```python
from build123d import *

# Parameters (mm, degrees)
SKETCH1_W             = 168
SKETCH1_H             = 89
BOSS_EXTRUDE1_DEPTH   = 70
SHELL1_T              = -0.8
F_8_0MM_DOWEL_HOLE1_D = 8


with BuildPart() as part:
    # Sketch1 → Boss-Extrude1 (new body)
    with BuildSketch(Plane(origin=(0, 0, 0), x_dir=(1, 0, 0), z_dir=(0, 1, 0))):
        Rectangle(SKETCH1_W, SKETCH1_H)
    extrude(amount=BOSS_EXTRUDE1_DEPTH)

    # Shell1
    shell1_openings = [part.faces().sort_by_distance(p)[0] for p in [
        (84, 35, 0),
    ]]
    offset(amount=SHELL1_T, openings=shell1_openings, kind=Kind.INTERSECTION)

    # Ø8.0mm Dowel Hole1 (through all)
    with Locations(Plane.XY.offset(44.5)):
        with Locations((64, 10), (-74, 60), (-64, 47.5), (-74, 35), (-64, 22.5), (-74, 10), (-54.285714286, 60), (-44.285714286, 47.5), (-54.285714286, 35), (-44.285714286, 22.5), (-54.285714286, 10), (-34.571428571, 60), (-24.571428571, 47.5), (-34.571428571, 35), (-24.571428571, 22.5), (-34.571428571, 10), (-14.857142857, 60), (-4.857142857, 47.5), (-14.857142857, 35), (-4.857142857, 22.5), (-14.857142857, 10), (4.857142857, 60), (14.857142857, 47.5), (4.857142857, 35), (14.857142857, 22.5), (4.857142857, 10), (24.571428571, 60), (34.571428571, 47.5), (24.571428571, 35), (34.571428571, 22.5), (24.571428571, 10), (44.285714286, 60), (54.285714286, 47.5), (44.285714286, 35), (54.285714286, 22.5), (44.285714286, 10), (64, 60), (74, 47.5), (64, 35), (74, 22.5)):
            Hole(F_8_0MM_DOWEL_HOLE1_D / 2)


solid = part.part
```
Can you work these out from the model? Positions are in its coordinate system, mm. A direction names the side the tool comes from. Coordinates: 2 decimals unless noted, no trailing zeros. Order: outer loops, then holes, each group sorted by start corner. A loop starts at its lowest first (then second) coordinate and runs counter-clockwise, first axis right, second up.
1. If we section it at B-B (x = 64): Give the number of separate pieces and of enclosed holes in the cut face, then the cut area to 3 significant figures.
2. For faces 1 (the face through (-73.479, 38.966, -44.106)), 2 (the face through (-83.2, 35, 1)), which set-ups out of +Z, -Z, +X, -X, +Y, -Y let a thin tool reach every point of the face, with its end or its side?
3. Thinking about a two-plate mould opening in Y: for faces 3 (the face through (-1, 70, -1)), 4 (the face through (-33.704, 56.095, 44.094)), which applies, +Y half, -Y half, draft (parallel to the pull), parting line (faces both ways), or undercut?
4. I'm going to push flat-ended pins straight in: pin 1 (5 mm diameter, centred on x = 24.57, y = 10, fed in from +Z); pin 2 (3 mm diameter, centred on y = 62.5, z = 29.5, fed in from +X). Where does each tip first touch, or does it pass through?
5. If we section it at D-D (x = -4): Please give me the cut outline in (y, z), then the cut area to 3 significant figures.
6. If we section it at A-A (x = -64): Please give me the cut outline in (y, z).
7. I need wall thicknesses on line 1 (Y direction, x = -64, z = -43.9); line 2 (Y direction, x = -3, z = 13); line 3 (Z direction, x = -55, y = 64). Which ranges of each line are inside material? Lowest first, please.
Entries:
1. separate pieces: 6
1. enclosed holes: 0
1. area: 213 mm2
2. face 1: +Z, -Z
2. face 2: +X
3. face 3: +Y half
3. face 4: undercut
4. pin 1: passes through
4. pin 2: stops at x = -83.2
5. outline: (0, -44.5) - (18.59, -44.5) - (18.59, -43.7) - (0.8, -43.7) - (0.8, 43.7) - (18.59, 43.7) - (18.59, 44.5) - (0, 44.5) - close; (26.41, -44.5) - (43.59, -44.5) - (43.59, -43.7) - (26.41, -43.7) - close; (26.41, 43.7) - (43.59, 43.7) - (43.59, 44.5) - (26.41, 44.5) - close; (51.41, -44.5) - (70, -44.5) - (70, 44.5) - (51.41, 44.5) - (51.41, 43.7) - (69.2, 43.7) - (69.2, -43.7) - (51.41, -43.7) - close
5. area: 227 mm2
6. outline: (0, -44.5) - (18.5, -44.5) - (18.5, -43.7) - (0.8, -43.7) - (0.8, 43.7) - (18.5, 43.7) - (18.5, 44.5) - (0, 44.5) - close; (26.5, -44.5) - (43.5, -44.5) - (43.5, -43.7) - (26.5, -43.7) - close; (26.5, 43.7) - (43.5, 43.7) - (43.5, 44.5) - (26.5, 44.5) - close; (51.5, -44.5) - (70, -44.5) - (70, 44.5) - (51.5, 44.5) - (51.5, 43.7) - (69.2, 43.7) - (69.2, -43.7) - (51.5, -43.7) - close
7. line 1: y = 0 to 18.5, 26.5 to 43.5, 51.5 to 70
7. line 2: y = 0 to 0.8, 69.2 to 70
7. line 3: z = -44.5 to -43.7, 43.7 to 44.5
